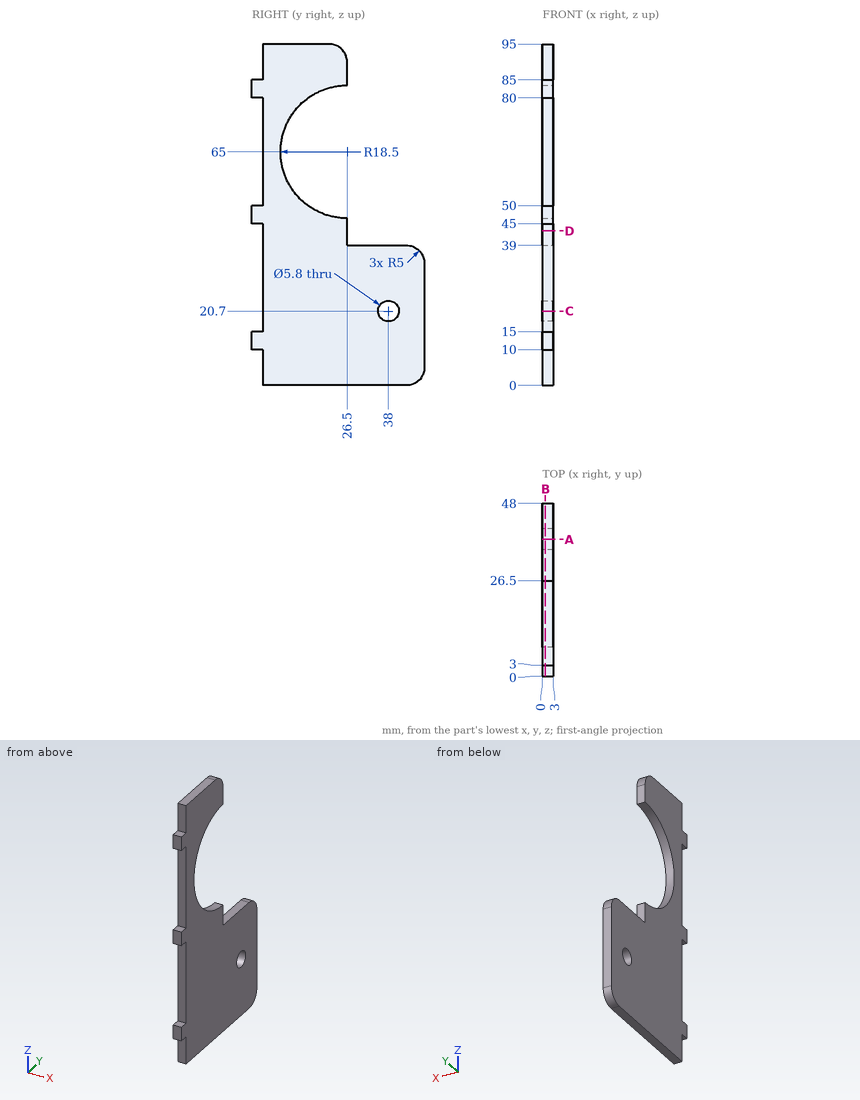
Check sheet for the drawn part. Datum: minimum x, y, z corner. Units: mm. Coordinates: 2 decimals unless noted, no trailing zeros. Loops run counter-clockwise (first coordinate to the right, second up) from the corner with the lowest first, then second, coordinate; pieces in that order, holes last. Notation, with made-up numbers: (62.5, 15.5) -> (115.5, 15.5) arc R11 ccw to (115.5, 27.5) -> close; hole circle Ø1 at (-11, 74). An arc over 180 degrees is marked (long way). Answer as CSV lines item,"result".
1) Depth check by flat-ended pin: pin 1 (0.9 mm diameter, centred on x = 1, z = 71.5, fed in from -Y); pin 2 (1.5 mm diameter, centred on x = 2, y = 1.5, fed in from +Z); pin 3 (0.9 mm diameter, centred on x = 2, y = 1, fed in from -Z). Enter the tip coordinate at first touch or a pass-through.
Found:
pin 1,"stops at y = 3"
pin 2,"stops at z = 85"
pin 3,"stops at z = 10"
2) Cross-section at A-A, the plane y = 38. Record the cut outline in (x, z).
Found:
outline,"(0, 0) -> (3, 0) -> (3, 17.8) -> (0, 17.8) -> close; (0, 23.6) -> (3, 23.6) -> (3, 39) -> (0, 39) -> close"
3) Thickness scan on L1, parallel to Y at x = 1.55, z = 20.7; L2, parallel to Y at x = 0.75, z = 88; L3, parallel to Z at x = 1.95, y = 15. Record the ranges inside material, lowest first. Write a range as from..to.
Found:
L1,"y = 3..35.1, 40.9..48"
L2,"y = 3..26.5"
L3,"z = 0..50.51, 79.49..95"
4) Cross-section at C-C, the plane z = 20.7. Record the cut outline in (x, y), then the cut area to 3 significant figures.
Found:
outline,"(0, 3) -> (3, 3) -> (3, 35.1) -> (0, 35.1) -> close; (0, 40.9) -> (3, 40.9) -> (3, 48) -> (0, 48) -> close"
area,"118 mm2"
5) Cross-section at D-D, the plane z = 43. Record the cut outline in (x, y), then the cut area to 3 significant figures.
Found:
outline,"(0, 3) -> (3, 3) -> (3, 26.5) -> (0, 26.5) -> close"
area,"70.5 mm2"
6) Cross-section at B-B, the plane x = 0.8. Record the cut outline in (y, z), then the cut area to 3 significant figures.
Found:
outline,"(0, 10) -> (3, 10) -> (3, 0) -> (43, 0) arc R5 ccw to (48, 5) -> (48, 34) arc R5 ccw to (43, 39) -> (26.5, 39) -> (26.5, 46.5) arc R18.5 cw to (26.5, 83.5) -> (26.5, 90) arc R5 ccw to (21.5, 95) -> (3, 95) -> (3, 85) -> (0, 85) -> (0, 80) -> (3, 80) -> (3, 50) -> (0, 50) -> (0, 45) -> (3, 45) -> (3, 15) -> (0, 15) -> close; hole circle Ø5.8 at (38, 20.7)"
area,"2,540 mm2"
